```python
from build123d import *

# Parameters (mm, degrees)
SKETCH1_W               = 60
SKETCH1_H               = 31.5
BOSS_EXTRUDE1_DEPTH     = 2
SKETCH2_W               = 60
SKETCH2_H               = 2
BOSS_EXTRUDE2_DEPTH     = 7
CUT_EXTRUDE1_DEPTH      = 45.0596187
CUT_EXTRUDE1_DEPTH_BACK = 45.0596187
SKETCH3_R               = 1.6
CHAMFER1_SIZE           = 3
CHAMFER3_SIZE           = 3
SKETCH4_R               = 1.25
SKETCH4_R_2             = 1.1
CUT_EXTRUDE2_DEPTH      = 10
SKETCH5_W               = 25.5
SKETCH5_H               = 3
CUT_EXTRUDE3_DEPTH      = 10


with BuildPart() as part:
    # Sketch1 → Boss-Extrude1 (new body)
    with BuildSketch(Plane(origin=(0, 0, 0), x_dir=(1, 0, 0), z_dir=(0, 1, 0))):
        Rectangle(SKETCH1_W, SKETCH1_H)
    extrude(amount=BOSS_EXTRUDE1_DEPTH)

    # Sketch2 → Boss-Extrude2 (add)
    with BuildSketch(Plane.XZ):
        with Locations((0, -14.75)):
            Rectangle(SKETCH2_W, SKETCH2_H)
        with Locations((0, 14.75)):
            Rectangle(SKETCH2_W, SKETCH2_H)
    extrude(amount=BOSS_EXTRUDE2_DEPTH)

    # Sketch3 → Cut-Extrude1 (cut, two sides: drawn at the far end of the back side and taken through both)
    with BuildSketch(Plane(origin=(0, 0, -15.75), x_dir=(-1, 0, 0), z_dir=(0, 0, -1)).offset(-CUT_EXTRUDE1_DEPTH_BACK)):
        with Locations((15, -4)):
            Circle(SKETCH3_R)
        with Locations(Location((-15, -4, 0), (0, 0, 180))):
            Circle(SKETCH3_R)
    extrude(amount=CUT_EXTRUDE1_DEPTH + CUT_EXTRUDE1_DEPTH_BACK, mode=Mode.SUBTRACT)

    # Chamfer1
    chamfer1_edges = [part.edges().sort_by_distance(p)[0] for p in [
        (30, -7, -14.75),
        (-30, -7, -14.75),
    ]]
    chamfer(chamfer1_edges, length=CHAMFER1_SIZE)

    # Chamfer3
    chamfer3_edges = [part.edges().sort_by_distance(p)[0] for p in [
        (30, -7, 14.75),
        (-30, -7, 14.75),
    ]]
    chamfer(chamfer3_edges, length=CHAMFER3_SIZE)

    # Sketch4 → Cut-Extrude2 (cut)
    with BuildSketch(Plane(origin=(0, 2, 0), x_dir=(1, 0, 0), z_dir=(0, 1, 0))):
        with Locations(Location((25.795, -5.801, 0), (0, 0, 270))):
            Circle(SKETCH4_R)
        with Locations(Location((4.205, -5.801, 0), (0, 0, 270))):
            Circle(SKETCH4_R)
        with Locations(Location((25.795, 9.439, 0), (0, 0, 270))):
            Circle(SKETCH4_R)
        with Locations(Location((4.205, 9.439, 0), (0, 0, 270))):
            Circle(SKETCH4_R)
        with Locations(Location((-26.335, -0.75, 0), (0, 0, 270))):
            Circle(SKETCH4_R_2)
        with Locations(Location((-26.335, 11.75, 0), (0, 0, 270))):
            Circle(SKETCH4_R_2)
        with Locations(Location((-5.335, -0.75, 0), (0, 0, 270))):
            Circle(SKETCH4_R_2)
        with Locations(Location((-5.335, 11.75, 0), (0, 0, 270))):
            Circle(SKETCH4_R_2)
    extrude(amount=-CUT_EXTRUDE2_DEPTH, mode=Mode.SUBTRACT)

    # Sketch5 → Cut-Extrude3 (cut)
    with BuildSketch(Plane.XZ):
        with Locations((-15.75, 12.25)):
            Rectangle(SKETCH5_W, SKETCH5_H)
    extrude(amount=-CUT_EXTRUDE3_DEPTH, mode=Mode.SUBTRACT)


solid = part.part
```
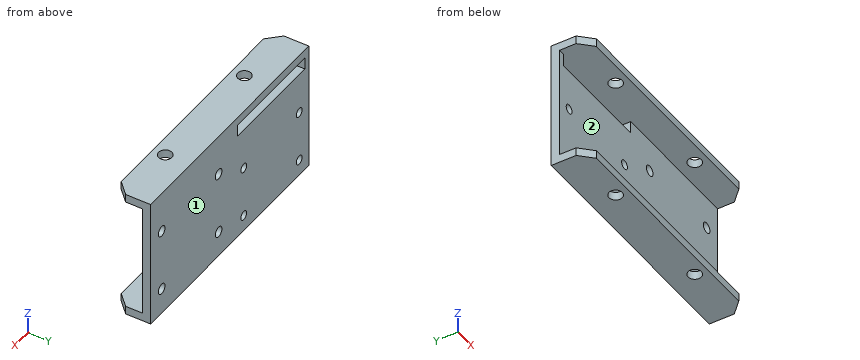
For this review, take the finished solid that the model builds, in its own axes (mm). Face numbers are marked on the shaded views. A direction names the side the tool comes from. Coordinates: 2 decimals unless noted, no trailing zeros. Order: outer loops, then holes, each group sorted by start corner. A loop starts at its lowest first (then second) coordinate and runs counter-clockwise, first axis right, second up. Notation, with made-up numbers: (-13.5, 38.5) - (9.5, 38.5) arc R6 cw to (9.5, 43.5) - close; hole circle Ø7 at (3, 0). An arc over 180 degrees is marked (long way). Answer as a JSON object with one key per item and string values. Group by question number.
1. We need section B-B on z = -11.75. State the section outline as (x, y) points (3 decimals), then the cut area to 3 significant figures.
2. For probe 1 along X at (y, z) = (0.8, 0.75) (3 decimals); probe 2 along Z at (x, y) = (15, -0.25); probe 3 along Y at (x, z) = (21, -9.5), list the stretches that pass through material, from the lowest coordinate up.
3. We need section A-A on x = -15. State the section outline as (y, z) points, then the cut area to 3 significant figures.
4. We need section D-D on x = 15. State the section outline as (y, z) points, then the cut area to 3 significant figures.
5. Clearance check with a flat-ended pin moving along its axis: P1, Ø3.5, axis at x = -5.335, z = -11.75, coming from the -Y side. State where the tip first meets the part, or that it passes through.
6. We need section C-C on y = -3. State the section outline as (x, z) points.
7. For the marked faces 1 and 2, list the 3-axis set-ups (+Z, -Z, +X, -X, +Y, -Y) from which the entire face can be reached by the end or side of a thin tool; tool diameter is ignored.
Final values:
{
 "1": {"outline": "(-30, 0) - (-27.435, 0) - (-27.435, 2) - (-30, 2) - close; (-25.235, 0) - (-6.435, 0) - (-6.435, 2) - (-25.235, 2) - close; (-4.235, 0) - (30, 0) - (30, 2) - (-4.235, 2) - close", "area": "111 mm²"},
 "2": {"probe 1": "-30 to -27.435, -25.235 to -6.435, -4.235 to 30", "probe 2": "-15.75 to -13.75, 13.75 to 15.75", "probe 3": "0 to 2"},
 "3": {"outline": "(-7, -15.75) - (-5.6, -15.75) - (-5.6, -13.75) - (-7, -13.75) - close; (-7, 13.75) - (-5.6, 13.75) - (-5.6, 15.75) - (-7, 15.75) - close; (-2.4, -15.75) - (2, -15.75) - (2, 10.75) - (0, 10.75) - (0, -13.75) - (-2.4, -13.75) - close; (-2.4, 13.75) - (2, 13.75) - (2, 15.75) - (-2.4, 15.75) - close", "area": "72.2 mm²"},
 "4": {"outline": "(-7, -15.75) - (-5.6, -15.75) - (-5.6, -13.75) - (-7, -13.75) - close; (-7, 13.75) - (-5.6, 13.75) - (-5.6, 15.75) - (-7, 15.75) - close; (-2.4, -15.75) - (2, -15.75) - (2, 15.75) - (-2.4, 15.75) - (-2.4, 13.75) - (0, 13.75) - (0, -13.75) - (-2.4, -13.75) - close", "area": "78.2 mm²"},
 "5": {"P1": "y = 0"},
 "6": {"outline": "(-30, -15.75) - (-16.25, -15.75) - (-16.25, -13.75) - (-30, -13.75) - close; (-30, 13.75) - (-16.25, 13.75) - (-16.25, 15.75) - (-30, 15.75) - close; (-13.75, -15.75) - (13.75, -15.75) - (13.75, -13.75) - (-13.75, -13.75) - close; (-13.75, 13.75) - (13.75, 13.75) - (13.75, 15.75) - (-13.75, 15.75) - close; (16.25, -15.75) - (30, -15.75) - (30, -13.75) - (16.25, -13.75) - close; (16.25, 13.75) - (30, 13.75) - (30, 15.75) - (16.25, 15.75) - close"},
 "7": {"face 1": "+Z, -Z, +X, -X, +Y", "face 2": "+X, -X, -Y"}
}
